from build123d import *

# Parameters (mm, degrees)
F0_R     = 11.615552
F1_DEPTH = 84.7
F2_R     = 7.202174
F3_DEPTH = 7.1
F4_R     = 4.202422
F5_DEPTH = 9.6
F6_R     = 3.379899
F7_SIZE  = 1.5


with BuildPart() as f1:
    # F0 (on Top) → F1 (new body)
    with BuildSketch(Plane.XY):
        Circle(F0_R)
    extrude(amount=F1_DEPTH)

    # F2 (on face) → F3 (join)
    with BuildSketch(Plane.XY.offset(84.7)):
        Circle(F2_R)
    extrude(amount=F3_DEPTH)

    # F4 (on face) → F5 (join)
    with BuildSketch(Plane.XY.offset(91.8)):
        Circle(F4_R)
    extrude(amount=F5_DEPTH)

    # F6
    f6_edges = [f1.edges().sort_by_distance(p)[0] for p in [
        (-11.615552, 0, 84.7),
    ]]
    fillet(f6_edges, radius=F6_R)

    # F7
    f7_edges = [f1.edges().sort_by_distance(p)[0] for p in [
        (-4.202422, 0, 101.4),
    ]]
    chamfer(f7_edges, length=F7_SIZE)


solid = f1.part
Model file for the job. Use its own axes, mm. A direction names the side the tool comes from. Round coordinates to 2 decimals unless told otherwise and drop trailing zeros. Loops run counter-clockwise (first coordinate to the right, second up) from the corner with the lowest first, then second, coordinate; pieces in that order, holes last. Notation, with made-up numbers: (-29, -22) - (4, -22) arc R37 ccw to (4, 17) - close; hole circle Ø3 at (35.5, 65). An arc over 180 degrees is marked (long way). Write each question's results on one line, items separated by ' | '.
(1) 3-axis set-ups, long thin cutter, end or side, ignore diameter. For faces 1 (the flat face through (3.1, -3.1, 91.8)), 2 (the flat face through (0, 0, 0)): which of +Z, -Z, +X, -X, +Y, -Y reach the whole face in a straight line?
Answer below:
face 1: +Z | face 2: -Z, +X, -X, +Y, -Y
(2) Wall check: L1, parallel to X at y = 0.5, z = 81; L2, parallel to Z at x = -1.25, y = 6.5; L3, parallel to X at y = -5.5, z = 85. Give the ranges that are in metal, low to high.
Answer below:
L1: x = -11.6 to 11.6 | L2: z = 0 to 91.8 | L3: x = -4.65 to 4.65
(3) Saw through at A-A, the plane x = 0. List the corners of the cut face in (y, z), then the cut area to 3 significant figures.
Answer below:
outline: (-11.62, 0) - (11.62, 0) - (11.62, 81.32) arc R3.38 ccw to (8.24, 84.7) - (7.2, 84.7) - (7.2, 91.8) - (4.2, 91.8) - (4.2, 99.9) - (2.7, 101.4) - (-2.7, 101.4) - (-4.2, 99.9) - (-4.2, 91.8) - (-7.2, 91.8) - (-7.2, 84.7) - (-8.24, 84.7) arc R3.38 ccw to (-11.62, 81.32) - close | area: 2,140 mm^2
(4) Pin check, flat tips, straight feed: pin 1 (1 mm diameter, centred on x = -3, z = 50.5, fed in from +Y); pin 2 (3 mm diameter, centred on y = 4, z = 84, fed in from -X); pin 3 (4 mm diameter, centred on y = -3.5, z = 74, fed in from -X). Stop position of each tip, or through.
Answer below:
pin 1: stops at y = 11.34 | pin 2: stops at x = -10.84 | pin 3: stops at x = -11.52
(5) Saw through at C-C, the plane z = 54. List the corners of the cut face in (x, y), then the cut area to 3 significant figures.
Answer below:
outline: circle Ø23.23 at (0, 0) | area: 424 mm^2
